Read the model definition and answer for the solid it produces. Units are mm, in the model's axes. A direction names the side the tool comes from. Round coordinates to 2 decimals unless told otherwise and drop trailing zeros. Order: outer loops, then holes, each group sorted by start corner. A loop starts at its lowest first (then second) coordinate and runs counter-clockwise, first axis right, second up. Notation, with made-up numbers: (26.5, 27) -> (48.5, 27) arc R21 cw to (48.5, 49) -> close; hole circle Ø1 at (16.5, 76.5). An arc over 180 degrees is marked (long way). One line per item, written item: value. Start each with the question number.
1. For faces 1 (the face through (0.3, 0.5, 47)), 2 (the face through (-26, 0, -1)), determine the directions among +Z, -Z, +X, -X, +Y, -Y from which every point of the face is accessible in a straight line to the end or side of a thin tool.
2. Section A-A (z = 0) is taken. Give the vertices of the cut face in (x, y).
3. Section C-C (x = 6.25) is taken. Give the vertices of the cut face in (y, z).
4. A flat-ended cylindrical pin translates along its axis: pin 1 Ø13 at (x, z) = (47.5, 0) entering from -Y. Find the tip coordinate at first contact, or state that the pin passes through.
5. The mould has two halves that part along Z. Classify faces 3 (the face through (-26, 1, -1)), 4 (the face through (47.22, 0.493, -13.486)), 5 (the face through (59, 0.5, -7.7)): released by +Z, released by -Z, zero draft, split by the parting line, or undercut.
6. Section B-B (y = 0.7) is taken. State how many separate pieces and enclosed holes the cut face has, then the cut area to 3 significant figures.
7. Section D-D (x = -6.25) is taken. Give the vertices of the cut face in (y, z), then the cut area to 3 significant figures.
8. Consider line 1 (X direction, y = 0.45, z = 0); line 2 (X direction, y = 0.85, z = -19); line 3 (X direction, y = 0.1, z = 28.5). Determine where each line is inside the solid, lowest interval first.
from build123d import *

# Parameters (mm, degrees)
SKETCH_1_R          = 59.5
SKETCH_1_R_2        = 25
SKETCH_1_R_3        = 1.6
EXTRUDE_1_DEPTH     = 1
SKETCH_2_R          = 8
SKETCH_2_R_2        = 7.5
CUT_EXTRUDE_1_DEPTH = 10


with BuildPart() as part:
    # 草图1 → 凸台-拉伸1 (new body)
    with BuildSketch(Plane(origin=(0, 0, 0), x_dir=(1, 0, 0), z_dir=(0, 1, 0))):
        with Locations(Location((0, 0, 0), (0, 0, 270))):
            Circle(SKETCH_1_R)
        with Locations(Location((0, 0, 0), (0, 0, 270))):
            Circle(SKETCH_1_R_2, mode=Mode.SUBTRACT)
        with Locations(Location((-6.25, 51.75, 0), (0, 0, 270))):
            Circle(SKETCH_1_R_3, mode=Mode.SUBTRACT)
        with Locations(Location((6.25, 51.75, 0), (0, 0, 270))):
            Circle(SKETCH_1_R_3, mode=Mode.SUBTRACT)
        with Locations(Location((6.25, -51.75, 0), (0, 0, 90))):
            Circle(SKETCH_1_R_3, mode=Mode.SUBTRACT)
        with Locations(Location((-6.25, -51.75, 0), (0, 0, 90))):
            Circle(SKETCH_1_R_3, mode=Mode.SUBTRACT)
        with BuildLine():
            ThreePointArc((49.880799132, 19.343109316), (46.332359102, 26.75), (41.692023621, 33.526484551))
            ThreePointArc((41.692023621, 33.526484551), (35.365233214, 34.213305594), (34.678412171, 27.886515187))
            ThreePointArc((34.678412171, 27.886515187), (38.538130468, 22.25), (41.489636661, 16.089128309))
            ThreePointArc((41.489636661, 16.089128309), (47.312208399, 13.520537577), (49.880799132, 19.343109316))
        make_face(mode=Mode.SUBTRACT)
        with BuildLine():
            ThreePointArc((41.692023621, -33.526484551), (46.332359102, -26.75), (49.880799132, -19.343109316))
            ThreePointArc((49.880799132, -19.343109316), (47.312208399, -13.520537577), (41.489636661, -16.089128309))
            ThreePointArc((41.489636661, -16.089128309), (38.538130468, -22.25), (34.678412171, -27.886515187))
            ThreePointArc((34.678412171, -27.886515187), (35.365233214, -34.213305594), (41.692023621, -33.526484551))
        make_face(mode=Mode.SUBTRACT)
        with BuildLine():
            ThreePointArc((-49.880799132, -19.343109316), (-46.332359102, -26.75), (-41.692023621, -33.526484551))
            ThreePointArc((-41.692023621, -33.526484551), (-35.365233214, -34.213305594), (-34.678412171, -27.886515187))
            ThreePointArc((-34.678412171, -27.886515187), (-38.538130468, -22.25), (-41.489636661, -16.089128309))
            ThreePointArc((-41.489636661, -16.089128309), (-47.312208399, -13.520537577), (-49.880799132, -19.343109316))
        make_face(mode=Mode.SUBTRACT)
        with BuildLine():
            ThreePointArc((-41.692023621, 33.526484551), (-46.332359102, 26.75), (-49.880799132, 19.343109316))
            ThreePointArc((-49.880799132, 19.343109316), (-47.312208399, 13.520537577), (-41.489636661, 16.089128309))
            ThreePointArc((-41.489636661, 16.089128309), (-38.538130468, 22.25), (-34.678412171, 27.886515187))
            ThreePointArc((-34.678412171, 27.886515187), (-35.365233214, 34.213305594), (-41.692023621, 33.526484551))
        make_face(mode=Mode.SUBTRACT)
    extrude(amount=EXTRUDE_1_DEPTH)

    # 草图2 → 切除-拉伸1 (cut)
    with BuildSketch(Plane.XZ):
        with Locations(Location((47.5, 0, 0), (0, 0, 270))):
            Circle(SKETCH_2_R)
        with Locations(Location((-47.5, 0, 0), (0, 0, 270))):
            Circle(SKETCH_2_R)
        with Locations(Location((-20.5, -42, 0), (0, 0, 270))):
            Circle(SKETCH_2_R_2)
        with BuildLine():
            ThreePointArc((4.096319909, -46.82115081), (16.074946736, -44.165553177), (26.958092508, -38.500146082))
            ThreePointArc((26.958092508, -38.500146082), (28.431546156, -30.143775198), (20.075175272, -28.67032155))
            ThreePointArc((20.075175272, -28.67032155), (11.970705016, -32.889241728), (3.050450996, -34.866814433))
            ThreePointArc((3.050450996, -34.866814433), (-2.403782736, -41.366917078), (4.096319909, -46.82115081))
        make_face()
        with BuildLine():
            ThreePointArc((23.5, 40.703193978), (0, 47), (-23.5, 40.703193978))
            ThreePointArc((-23.5, 40.703193978), (-25.696152423, 32.507041555), (-17.5, 30.310889132))
            ThreePointArc((-17.5, 30.310889132), (0, 35), (17.5, 30.310889132))
            ThreePointArc((17.5, 30.310889132), (25.696152423, 32.507041555), (23.5, 40.703193978))
        make_face()
    extrude(amount=-CUT_EXTRUDE_1_DEPTH, mode=Mode.SUBTRACT)


solid = part.part
Answer:
1. face 1: +Y, -Y
1. face 2: +Z, -Z, +X, -X, -Y
2. outline: (-59.5, 0) -> (-55.5, 0) -> (-55.5, 1) -> (-59.5, 1) -> close; (-39.5, 0) -> (-25, 0) -> (-25, 1) -> (-39.5, 1) -> close; (25, 0) -> (39.5, 0) -> (39.5, 1) -> (25, 1) -> close; (55.5, 0) -> (59.5, 0) -> (59.5, 1) -> (55.5, 1) -> close
3. outline: (0, -59.17) -> (1, -59.17) -> (1, -53.35) -> (0, -53.35) -> close; (0, -50.15) -> (1, -50.15) -> (1, -46.58) -> (0, -46.58) -> close; (0, -34.44) -> (1, -34.44) -> (1, -24.21) -> (0, -24.21) -> close; (0, 24.21) -> (1, 24.21) -> (1, 34.44) -> (0, 34.44) -> close; (0, 46.58) -> (1, 46.58) -> (1, 50.15) -> (0, 50.15) -> close; (0, 53.35) -> (1, 53.35) -> (1, 59.17) -> (0, 59.17) -> close
4. pin 1: through
5. face 3: zero draft
5. face 4: undercut
5. face 5: split by the parting line
6. separate pieces: 1
6. enclosed holes: 14
6. area: 6,750 mm^2
7. outline: (0, -59.17) -> (1, -59.17) -> (1, -53.35) -> (0, -53.35) -> close; (0, -50.15) -> (1, -50.15) -> (1, -24.21) -> (0, -24.21) -> close; (0, 24.21) -> (1, 24.21) -> (1, 34.44) -> (0, 34.44) -> close; (0, 46.58) -> (1, 46.58) -> (1, 50.15) -> (0, 50.15) -> close; (0, 53.35) -> (1, 53.35) -> (1, 59.17) -> (0, 59.17) -> close
7. area: 51.4 mm^2
8. line 1: -59.5 to -55.5, -39.5 to -25, 25 to 39.5, 55.5 to 59.5
8. line 2: -56.38 to -50, -40.24 to -16.25, 16.25 to 40.24, 50 to 56.38
8. line 3: -52.23 to -45.28, -34.26 to 34.26, 45.28 to 52.23
